from build123d import *

# Parameters (mm, degrees)
ESTRUSIONE_ESTRUSIONE1_DEPTH                         = 35
ESTRUSIONE_ESTRUSIONE2_DEPTH                         = 22
ESTRUSIONE_ESTRUSIONE3_DEPTH                         = 20
TAGLIO_ESTRUSIONE1_DEPTH                             = 111.588362117
TAGLIO_ESTRUSIONE1_DEPTH_BACK                        = 111.588362117
SCHIZZO3_W                                           = 30
SCHIZZO3_H                                           = 5
FORO_22_0_22_1_D                                     = 22
FORO_LAMATO_PER_VITE_M10_A_TESTA_CILINDR_D           = 11
FORO_LAMATO_PER_VITE_M10_A_TESTA_CILINDR_CBORE_D     = 18
FORO_LAMATO_PER_VITE_M10_A_TESTA_CILINDR_CBORE_DEPTH = 10.6
FORO_16_0_16_1_D                                     = 16
RACCORDO1_R                                          = 22


with BuildPart() as part:
    # Schizzo1 → Estrusione-Estrusione1 (new, symmetric)
    with BuildSketch(Plane(origin=(0, 0, 0), x_dir=(0, 0, -1), z_dir=(1, 0, 0))):
        Polygon((0, 0), (0, 20), (-25, 20), (-35, 20), (-35, 0), align=None)
        Polygon((25, 20), (0, 20), (0, 0), (35, 0), (35, 20), align=None)
    extrude(amount=ESTRUSIONE_ESTRUSIONE1_DEPTH, both=True)

    # Schizzo1<3> → Estrusione-Estrusione2 (add, symmetric)
    with BuildSketch(Plane(origin=(0, 0, 0), x_dir=(0, 0, -1), z_dir=(1, 0, 0))):
        Polygon((0, 20), (0, 30), (-10, 30), (-10, 70), (-25, 70), (-25, 20), align=None)
        Polygon((10, 30), (0, 30), (0, 20), (25, 20), (25, 70), (10, 70), align=None)
    extrude(amount=ESTRUSIONE_ESTRUSIONE2_DEPTH, both=True)

    # Schizzo2 → Estrusione-Estrusione3 (add)
    with BuildSketch(Plane.XZ):
        with BuildLine():
            Line((-35, 35), (-35, -35))
            ThreePointArc((-35, -35), (-49.292857857, 0), (-35, 35))
        make_face()
        with BuildLine():
            Line((35, 35), (35, -35))
            ThreePointArc((35, -35), (49.292857857, 0), (35, 35))
        make_face()
    extrude(amount=-ESTRUSIONE_ESTRUSIONE3_DEPTH)

    # Schizzo3 → Taglio-Estrusione1 (cut, two sides: drawn at the far end of the back side and taken through both)
    with BuildSketch(Plane(origin=(0, 0, -35), x_dir=(-1, 0, 0), z_dir=(0, 0, -1)).offset(-TAGLIO_ESTRUSIONE1_DEPTH_BACK)):
        with Locations((0, 2.5)):
            Rectangle(SCHIZZO3_W, SCHIZZO3_H)
    extrude(amount=TAGLIO_ESTRUSIONE1_DEPTH + TAGLIO_ESTRUSIONE1_DEPTH_BACK, mode=Mode.SUBTRACT)

    # Foro Ø22.0 (22)-1 (through all)
    with Locations(Plane.XY.offset(25)):
        with Locations((0, 48)):
            Hole(FORO_22_0_22_1_D / 2)

    # Foro lamato per Vite M10 a testa cilindrica-1 (through all)
    with Locations(Plane(origin=(0, 20, 0), x_dir=(1, 0, 0), z_dir=(0, 1, 0))):
        with Locations((35, 0), (-35, 0)):
            CounterBoreHole(FORO_LAMATO_PER_VITE_M10_A_TESTA_CILINDR_D / 2, FORO_LAMATO_PER_VITE_M10_A_TESTA_CILINDR_CBORE_D / 2, FORO_LAMATO_PER_VITE_M10_A_TESTA_CILINDR_CBORE_DEPTH)

    # Foro Ø16.0 (16)-1 (through all)
    with Locations(Plane(origin=(0, 30, 0), x_dir=(1, 0, 0), z_dir=(0, 1, 0))):
        with Locations((0, 0)):
            Hole(FORO_16_0_16_1_D / 2)

    # Raccordo1
    raccordo1_edges = [part.edges().sort_by_distance(p)[0] for p in [
        (-22, 70, 17.5),
        (22, 70, 17.5),
        (-22, 70, -17.5),
        (22, 70, -17.5),
    ]]
    fillet(raccordo1_edges, radius=RACCORDO1_R - 0.0001)  # a hair under: the kernel refuses the full size


solid = part.part
Source: CAD feature listing. Evaluate the final solid. Frame: model axes, mm. A direction names the side the tool comes from. Give positions to 0.01 mm unless a question says otherwise; leave off trailing zeros. Loops run counter-clockwise (first coordinate to the right, second up) from the corner with the lowest first, then second, coordinate; pieces in that order, holes last. Notation, with made-up numbers: (-0.5, -6) -> (53.5, -6) arc R22 ccw to (53.5, 0) -> close; hole circle Ø2 at (67, 79.25). An arc over 180 degrees is marked (long way). Use a Markdown table: item, result. Add a question column.
1) Section query D-D, the plane y = 13.5. Return the cut outline in (x, z), then the cut area to 3 significant figures.
2) Section query B-B, the plane z = 0. Count the separate pieces of the cut face and the enclosed holes in it, then the cut area to 3 significant figures.
3) Section query A-A, the plane y = 34. Return the cut outline in (x, z).
4) Section query C-C, the plane x = 37. Return the cut outline in (y, z), then the cut area to 3 significant figures.
5) Line query: line 1 along Y through (x, z) = (0, 20); line 2 along Z through (x, y) = (0, 20.25); line 3 along Z through (x, y) = (-35, 3). Output: solid intervals per line, ascending. Write a range as [from, to].
6) First-contact query: pin 1 (9 mm diameter, centred on x = -34.5, z = 1, fed in from +Y); pin 2 (12 mm diameter, centred on x = -10.5, y = 53, fed in from -Z); pin 3 (8 mm diameter, centred on y = 33, z = 19, fed in from +X); pin 4 (20 mm diameter, centred on x = 0, y = 48, fed in from -Z). Flat tips, straight axial feed; report the tip coordinate or a pass-through.
7) Pull-direction query (X, two-part tool) for faces 5 (the face through (49.29, 9.86, -0.54)), 6 (the face through (-15.73, 63.38, 17.6)), 7 (the face through (0, 10, 35)), 8 (the face through (-31, 9.4, -4)); classes: +X half, -X half, draft (parallel to the pull), parting line (faces both ways), or undercut.
8) Reachability of faces 1 (the face through (15, 2, 0)), 2 (the face through (0, 34, -25)), 3 (the face through (5, 30, -7)), 4 (the face through (39, 9.4, -4)) from +Z, -Z, +X, -X, +Y, -Y: full face, straight path, thin tool, end or side. Return the list, or none.
Numbers:
| question | item | result |
|---|---|---|
| 1 | outline | (-35, -35) -> (35, -35) arc R50 ccw to (35, 35) -> (-35, 35) arc R50 ccw to start; hole circle Ø18 at (-35, 0); hole circle Ø16 at (0, 0); hole circle Ø18 at (35, 0) |
| 1 | area | 5,570 mm2 |
| 2 | separate pieces | 4 |
| 2 | enclosed holes | 0 |
| 2 | area | 1,270 mm2 |
| 3 | outline | (-22, -25) -> (22, -25) -> (22, -10) -> (-22, -10) -> close; (-22, 10) -> (22, 10) -> (22, 25) -> (-22, 25) -> close |
| 4 | outline | (0, -32.84) -> (20, -32.84) -> (20, -8.77) -> (9.4, -8.77) -> (9.4, -5.12) -> (0, -5.12) -> close; (0, 5.12) -> (9.4, 5.12) -> (9.4, 8.77) -> (20, 8.77) -> (20, 32.84) -> (0, 32.84) -> close |
| 4 | area | 1,030 mm2 |
| 5 | line 1 | y = [5, 37], [59, 70] |
| 5 | line 2 | z = [-25, -8], [8, 25] |
| 5 | line 3 | z = [-35, -5.5], [5.5, 35] |
| 6 | pin 1 | stops at y = 9.4 |
| 6 | pin 2 | stops at z = -25 |
| 6 | pin 3 | stops at x = 22 |
| 6 | pin 4 | passes through |
| 7 | face 5 | +X half |
| 7 | face 6 | -X half |
| 7 | face 7 | draft |
| 7 | face 8 | undercut |
| 8 | face 1 | +Z, -Z, -Y |
| 8 | face 2 | -Z, +X, -X, +Y |
| 8 | face 3 | +X, -X, +Y |
| 8 | face 4 | +Y |
